Can you work these out from the drawing? Everything is in mm from the part's minimum corner. Round coordinates to 2 decimals unless told otherwise and drop trailing zeros. Write each loop counter-clockwise with the first axis right and the second up, starting at its lowest first coordinate (ties: lowest second). Pieces come first, ordered by that corner, then holes. Notation, with made-up numbers: (-5.5, 54.25) - (-0.5, 54.25) arc R23 ccw to (-0.5, 75.25) - close; hole circle Ø2 at (-24, 77.5). An arc over 180 degrees is marked (long way). Write each question's results on one line, items separated by ' | '. Start each with the question number.
(1) Imagine slicing it at B-B on y = 12. Write out the boundary of the cut face in (x, z), then the cut area to 3 significant figures.
(2) Imagine slicing it at D-D on y = 2.5. Write out the boundary of the cut face in (x, z).
(3) For P1, Ø2, axis at y = 18, z = 22.5, coming from the +X side; P2, Ø12, axis at y = 3.5, z = 14.5, coming from the +X side, each with a flat end and sliding along its axis, tell me the tip position at first contact or that it passes through.
(4) Imagine slicing it at C-C on x = 11. Write out the boundary of the cut face in (y, z).
(5) Please list where these lines run through material, in increasing order: line 1 (X direction, y = 15, z = 3.25); line 2 (Y direction, x = 18.75, z = 22.25) (1 decimal); line 3 (Y direction, x = 19.5, z = 13.5) (1 decimal). Write a range as [from, to].
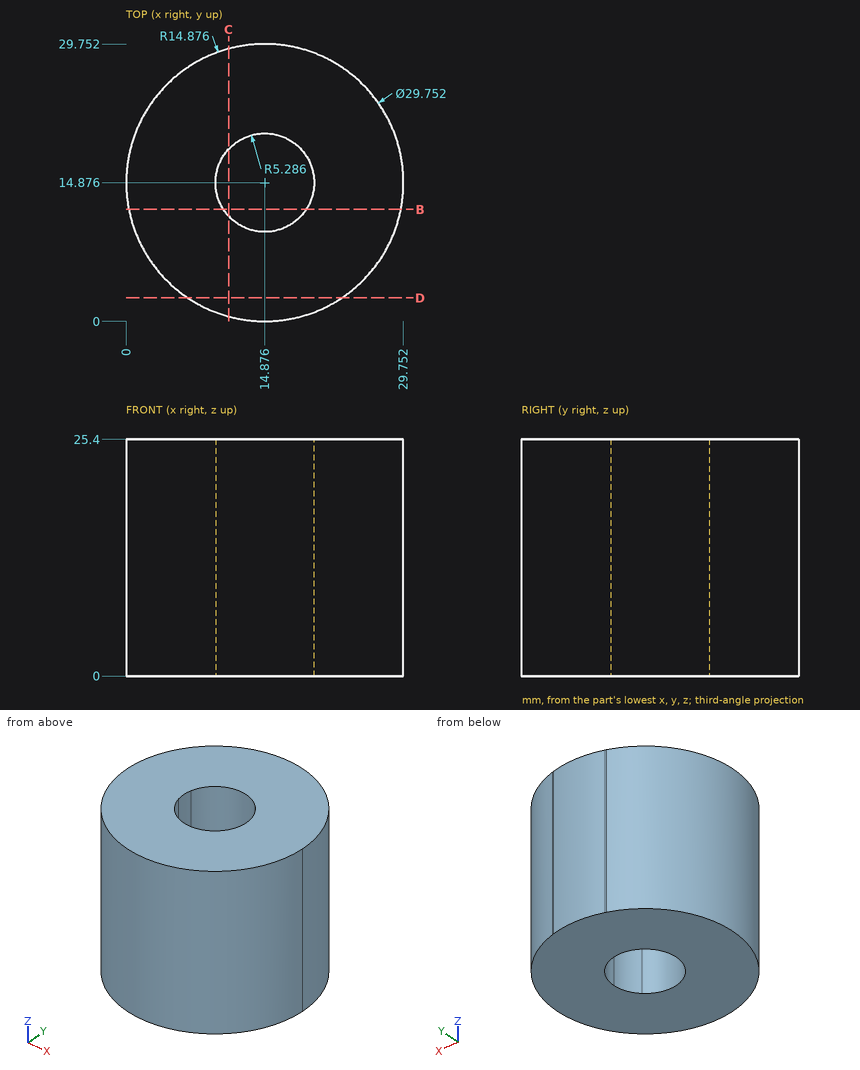
Response:
1) outline: (0.28, 0) - (10.44, 0) - (10.44, 25.4) - (0.28, 25.4) - close; (19.31, 0) - (29.47, 0) - (29.47, 25.4) - (19.31, 25.4) - close | area: 516 mm²
2) outline: (6.62, 0) - (23.13, 0) - (23.13, 25.4) - (6.62, 25.4) - close
3) P1: x = 29.6 | P2: x = 28.75
4) outline: (0.51, 0) - (11.28, 0) - (11.28, 25.4) - (0.51, 25.4) - close; (18.47, 0) - (29.24, 0) - (29.24, 25.4) - (18.47, 25.4) - close
5) line 1: [0, 9.59], [20.16, 29.75] | line 2: [0.5, 11.3], [18.5, 29.2] | line 3: [0.7, 12.3], [17.4, 29]
